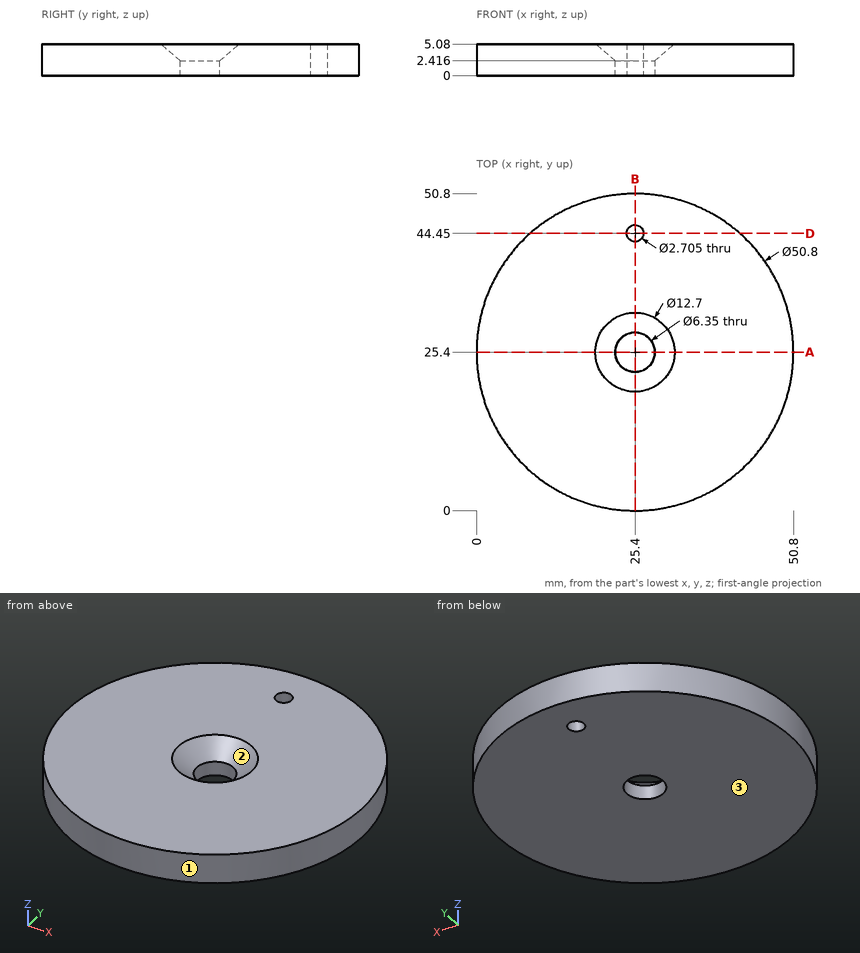
Geometry: see drawing. Coordinates: mm, zero at the bounding-box minimum. Give positions to 0.01 mm unless a question says otherwise; leave off trailing zeros. Loops run counter-clockwise (first coordinate to the right, second up) from the corner with the lowest first, then second, coordinate; pieces in that order, holes last. Notation, with made-up numbers: M 68.5,41.5 L 96.5,41.5 A20 cw 96.5,53.5 Z; hole C 87.5,8.25 d9. An arc over 180 degrees is marked long. Answer as CSV lines item,"result". Start each with the question number.
1. Section B-B on x = 25.4. State how many separate pieces and enclosed holes the cut face has, plus the area to 3 significant figures.
2. Section A-A on y = 25.4. Return loops of the section in (x, z) (3 decimals), plus the area to 3 significant figures.
3. Pull-direction query (Y, two-part tool) for the marked faces 1, 2 and 3; classes: released by +Y, released by -Y, zero draft, split by the parting line, or undercut.
4. Section D-D on y = 44.45. Return loops of the section in (x, z).
5. Pin query (flat end, axial travel): P1, Ø3, axis at x = 11.5, z = 4.5, coming from the -Y side; P2, Ø1.5, axis at y = 9.5, z = 4, coming from the -X side; P3, Ø1, axis at x = 33.5, z = 3, coming from the +Y side. Return the tip coordinate at first contact, or that it passes through.
6. Line query: L1, parallel to Y at x = 25.4, z = 2.4 (1 decimal); L2, parallel to Y at x = 25.4, z = 2.9; L3, parallel to X at y = 28, z = 1.1. Output: solid intervals per line, ascending.
Computed values:
1,separate pieces,"3"
1,enclosed holes,"0"
1,area,"204 mm²"
2,outline,"M 0,0 L 22.225,0 L 22.225,2.416 L 19.05,5.08 L 0,5.08 Z; M 28.575,0 L 50.8,0 L 50.8,5.08 L 31.75,5.08 L 28.575,2.416 Z"
2,area,"217 mm²"
3,face 1,"split by the parting line"
3,face 2,"undercut"
3,face 3,"zero draft"
4,outline,"M 8.6,0 L 24.05,0 L 24.05,5.08 L 8.6,5.08 Z; M 26.75,0 L 42.2,0 L 42.2,5.08 L 26.75,5.08 Z"
5,P1,"stops at y = 3.23"
5,P2,"stops at x = 5.01"
5,P3,"stops at y = 49.64"
6,L1,"y = 0 to 22.2, 28.6 to 43.1, 45.8 to 50.8"
6,L2,"y = 0 to 21.65, 29.15 to 43.1, 45.8 to 50.8"
6,L3,"x = 0.13 to 23.58, 27.22 to 50.67"
